Work out the finished part from the listing and answer in its coordinate system (mm). Face numbers are marked on the shaded views. Give positions to 0.01 mm unless a question says otherwise; leave off trailing zeros. Loops run counter-clockwise (first coordinate to the right, second up) from the corner with the lowest first, then second, coordinate; pieces in that order, holes last. Notation, with made-up numbers: (60.5, 56) - (107.5, 56) arc R6 ccw to (107.5, 61) - close; hole circle Ø2 at (49.5, 6). An arc over 180 degrees is marked (long way). One line per question, with ' | ' between items.
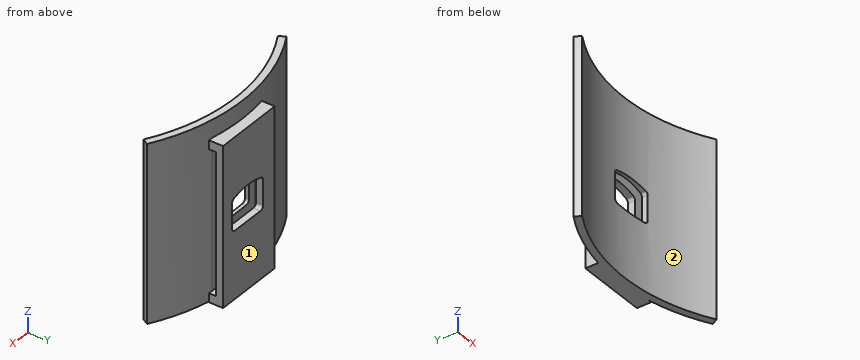
from build123d import *

# Parameters (mm, degrees)
BOX002_W                    = 20
BOX002_H                    = 2
BOX002_DEPTH                = 40
EXTRUDE_DEPTH               = 6
EXTRUDE001_DEPTH            = 6
THICKNESS_T                 = 1
BOX001_W                    = 20
BOX001_H                    = 4
BOX001_DEPTH                = 45
CYLINDER001_W               = 52
CYLINDER001_H               = 50
CYLINDER001_ANGLE           = 60
CYLINDER001_PLACEMENT_ANGLE = 60
CYLINDER_W                  = 54
CYLINDER_H                  = 50
CYLINDER_ANGLE              = 60
CYLINDER_PLACEMENT_ANGLE    = 60


with BuildPart() as slot:
    # Box002 → Box002 (new body)
    with BuildSketch(Plane(origin=(2, 44, 2.5), x_dir=(1, 0, 0), z_dir=(0, 0, 1))):
        with Locations((10, 1)):
            Rectangle(BOX002_W, BOX002_H)
    extrude(amount=BOX002_DEPTH)


with BuildPart() as extrude_body:
    with BuildSketch(Plane(origin=(8.5, 45, 6), x_dir=(1, 0, 0), z_dir=(0, 1, 0))):
        with BuildLine():
            Line((5, 4), (-5, 4))
            Line((-5, 4), (-5, -3.142136))
            ThreePointArc((-5, -3.142136), (-2.53653, -3.783978), (0, -4))
            ThreePointArc((0, -4), (2.53653, -3.783978), (5, -3.142136))
            Line((5, -3.142136), (5, 4))
        make_face()
    extrude(amount=EXTRUDE_DEPTH)


with BuildPart() as extrude001:
    with BuildSketch(Plane(origin=(8.5, 45, 6), x_dir=(1, 0, 0), z_dir=(0, 1, 0))):
        with BuildLine():
            Line((5, 4), (-5, 4))
            Line((-5, 4), (-5, -3.142136))
            ThreePointArc((-5, -3.142136), (-2.53653, -3.783978), (0, -4))
            ThreePointArc((0, -4), (2.53653, -3.783978), (5, -3.142136))
            Line((5, -3.142136), (5, 4))
        make_face()
    extrude(amount=EXTRUDE001_DEPTH)


with BuildPart() as pin_opening:
    # Thickness base: copy of Extrude body
    add(extrude_body.part)

    # Thickness
    thickness_openings = [pin_opening.faces().sort_by_distance(p)[0] for p in [
        (8.5, 51, 5.862901),
    ]]
    offset(amount=THICKNESS_T, openings=thickness_openings)

    # Fusion002: union Extrude body, Extrude001
    add(extrude_body.part)
    add(extrude001.part)


with BuildPart() as pin_opening_1:
    # Fusion002 placement: moved
    add(pin_opening.part.moved(Location((2, -3, 18))))


with BuildPart() as latch:
    # Box001 → Box001 (new body)
    with BuildSketch(Plane(origin=(0, 44, 0), x_dir=(1, 0, 0), z_dir=(0, 0, 1))):
        with Locations((10, 2)):
            Rectangle(BOX001_W, BOX001_H)
    extrude(amount=BOX001_DEPTH)


with BuildPart() as bottle_wall001:
    # Cylinder001 → Cylinder001 (revolve)
    with BuildSketch(Plane.XZ):
        with Locations((26, 25)):
            Rectangle(CYLINDER001_W, CYLINDER001_H)
    revolve(axis=Axis((0, 0, 0), (0, 0, 1)), revolution_arc=CYLINDER001_ANGLE)


with BuildPart() as bottle_wall001_1:
    # Cylinder001 placement: moved
    add(bottle_wall001.part.moved(Location((8.5, -7, 0))).rotate(Axis((8.5, -7, 0), (0, 0, 1)), CYLINDER001_PLACEMENT_ANGLE))


with BuildPart() as cut004:
    # Cylinder → Cylinder (revolve)
    with BuildSketch(Plane.XZ):
        with Locations((27, 25)):
            Rectangle(CYLINDER_W, CYLINDER_H)
    revolve(axis=Axis((0, 0, 0), (0, 0, 1)), revolution_arc=CYLINDER_ANGLE)


with BuildPart() as cut004_1:
    # Cylinder placement: moved
    add(cut004.part.moved(Location((8.5, -7, 0))).rotate(Axis((8.5, -7, 0), (0, 0, 1)), CYLINDER_PLACEMENT_ANGLE))

    # Cut: cut bottle_wall001
    add(bottle_wall001_1.part, mode=Mode.SUBTRACT)


with BuildPart() as cut004_2:
    # Cut placement: moved
    add(cut004_1.part.moved(Location((0, -2, 0))))

    # Fusion: union latch
    add(latch.part)

    # Fusion001: union latch
    add(latch.part)

    # Cut003: cut pin opening
    add(pin_opening_1.part, mode=Mode.SUBTRACT)

    # Cut004: cut slot
    add(slot.part, mode=Mode.SUBTRACT)


solid = cut004_2.part
1. Find section D-D on z = 14. Write down the section's boundary in (x, y).
Evaluation:
outline: (-18.5, 37.77) - (-17.5, 36.03) arc R52 cw to (34.5, 36.03) - (35.5, 37.77) arc R54 ccw to (18.84, 44) - (2, 44) - (2, 46) - (20, 46) - (20, 48) - (0, 48) - (0, 44.33) arc R54 ccw to start
2. Flat-ended cylindrical pins translate along their axes: pin 1 (1.5 mm diameter, centred on x = -10.5, z = 38.5, fed in from -Y); pin 2 (2 mm diameter, centred on y = 42, z = 38, fed in from -X); pin 3 (2 mm diameter, centred on x = -12, z = 32.5, fed in from -Y). Find the tip coordinate at first contact, or state that the pin passes through.
Evaluation:
pin 1: y = 39.1 | pin 2: x = -11.9 | pin 3: y = 38.35
3. Find section A-A on z = 23.5. Write down the section's boundary in (x, y), then the cut area to 3 significant figures.
Evaluation:
outline: (-18.5, 37.77) - (-17.5, 36.03) arc R52 cw to (4.5, 42.85) - (4.5, 44) - (2, 44) - (2, 46) - (4.5, 46) - (4.5, 48) - (0, 48) - (0, 44.33) arc R54 ccw to start; (16.5, 42.38) arc R52 cw to (34.5, 36.03) - (35.5, 37.77) arc R54 ccw to (18.84, 44) - (16.5, 44) - close; (16.5, 46) - (20, 46) - (20, 48) - (16.5, 48) - close | area: 104 mm2
4. Determine the mould class of the marked faces 1 and 2 for opening direction X: +X half, -X half, draft (parallel to the pull), parting line (faces both ways), or undercut.
Evaluation:
face 1: draft | face 2: undercut
5. Find section C-C on x = 6.5. Write down the section's boundary in (y, z).
Evaluation:
outline: (42.96, 0) - (48, 0) - (48, 19) - (46, 19) - (46, 2.5) - (44, 2.5) - (44, 19) - (42.96, 19) - close; (42.96, 28.49) - (44, 28.49) - (44, 42.5) - (46, 42.5) - (46, 28.49) - (48, 28.49) - (48, 45) - (44.96, 45) - (44.96, 50) - (42.96, 50) - close
6. Consider L1, parallel to Y at x = 12.5, z = 18; L2, parallel to Z at x = 18, y = 44.5; L3, parallel to X at y = 47, z = 12. Determine where each line is inside the solid, lowest interval first.
Evaluation:
L1: 42.85 to 44, 46 to 48 | L2: 0 to 2.5, 42.5 to 45 | L3: 0 to 20
